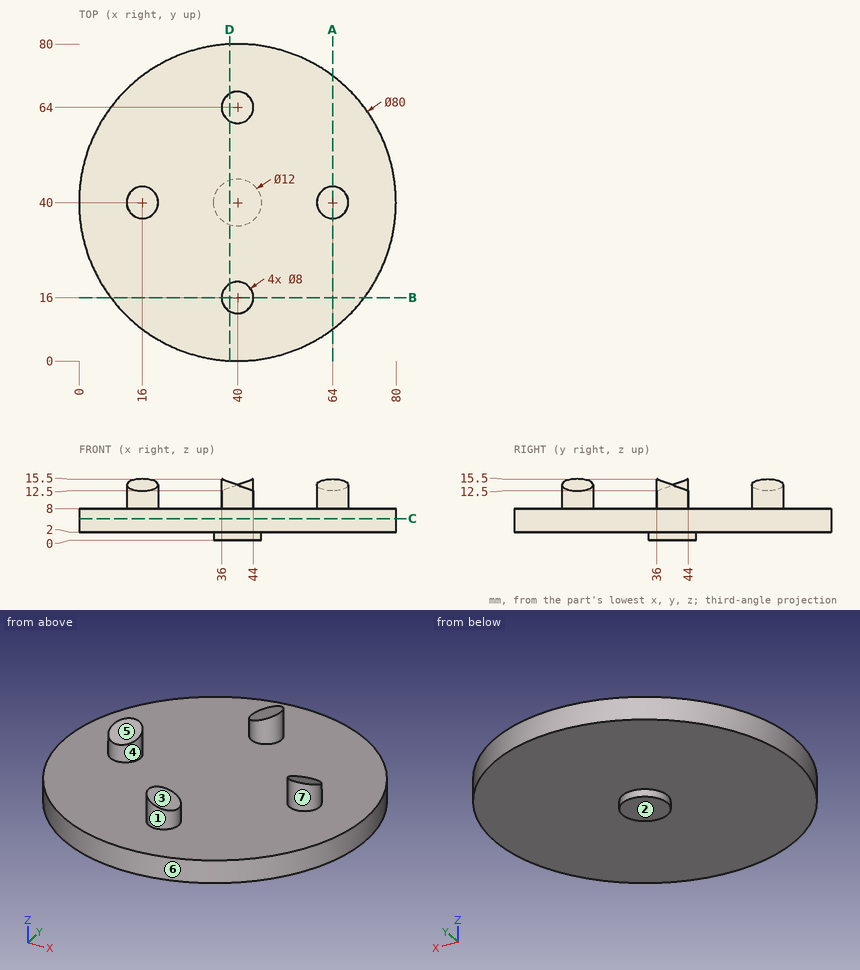
Check sheet for the drawn part. Datum: minimum x, y, z corner. Units: mm. A direction names the side the tool comes from. Give positions to 0.01 mm unless a question says otherwise; leave off trailing zeros. Loops run counter-clockwise (first coordinate to the right, second up) from the corner with the lowest first, then second, coordinate; pieces in that order, holes last.
1) Sectioned sample at A-A, the plane x = 64. Enter the section's corners in (y, z), then the cut area to 3 significant figures.
2) Set-up check for the marked faces 1, 2 and 3: record each of +Z, -Z, +X, -X, +Y, -Y from which the full face is reachable in a straight line by a thin tool's end or side.
3) Depth check by flat-ended pin: pin 1 Ø5 at (y, z) = (65.5, 8) entering from +X; pin 2 Ø12 at (x, y) = (49, 25) entering from -Z; pin 3 Ø5 at (x, z) = (29, 3.5) entering from -Y; pin 4 Ø2 at (x, z) = (22, 11.5) entering from -Y. Enter the tip coordinate at first touch or a pass-through.
4) Thickness scan on line 1 along Z through (x, y) = (36.5, 58.5); line 2 along Z through (x, y) = (41, 34.5); line 3 along X through (y, z) = (73, 7.5). Record the ranges inside material, lowest first.
5) Draft check along X on the marked faces 4, 5, 6 and 7. Enter one of: pulls with the +X half, pulls with the -X half, needs draft (parallel to the pull), parting line crosses it, or undercut.
6) Sectioned sample at C-C, the plane z = 5.5. Enter the section's corners in (x, y).
7) Sectioned sample at D-D, the plane x = 38. Enter the section's corners in (y, z).
Answers:
1. outline: (8, 2) - (72, 2) - (72, 8) - (44, 8) - (44, 12.5) - (36, 15.5) - (36, 8) - (8, 8) - close
1. area: 432 mm2
2. face 1: +Z
2. face 2: -Z, +X, -X, +Y, -Y
2. face 3: +Z, +X, -Y
3. pin 1: stops at x = 72.73
3. pin 2: stops at z = 2
3. pin 3: stops at y = 0.91
3. pin 4: passes through
4. line 1: z = 2 to 8
4. line 2: z = 0 to 8
4. line 3: x = 17.39 to 62.61
5. face 4: undercut
5. face 5: needs draft
5. face 6: parting line crosses it
5. face 7: undercut
6. outline: circle Ø80 at (40, 40)
7. outline: (0.05, 2) - (34.34, 2) - (34.34, 0) - (45.66, 0) - (45.66, 2) - (79.95, 2) - (79.95, 8) - (67.46, 8) - (67.46, 13.25) - (60.54, 13.25) - (60.54, 8) - (19.46, 8) - (19.46, 14.75) - (12.54, 14.75) - (12.54, 8) - (0.05, 8) - close
